from build123d import *

# Parameters (mm, degrees)
F0_R      = 16.5
F1_DEPTH  = 9.4
F2_R      = 14
F3_DEPTH  = 7.62
F4_R      = 2
F6_DEPTH  = 7
F8_DEPTH  = 5.5
F9_R      = 1
F10_R     = 10
F11_DEPTH = 3


with BuildPart() as f1:
    # F0 (on Top) → F1 (new body)
    with BuildSketch(Plane.XY):
        Circle(F0_R)
    extrude(amount=F1_DEPTH)

    # F2 (on face) → F3 (cut)
    with BuildSketch(Plane.XY.offset(9.4)):
        Circle(F2_R)
    extrude(amount=-F3_DEPTH, mode=Mode.SUBTRACT)

    # F4
    f4_edges = [f1.edges().sort_by_distance(p)[0] for p in [
        (-16.5, 0, 9.4),
    ]]
    fillet(f4_edges, radius=F4_R)

    # F5 (on face) → F6 (cut)
    with BuildSketch(Plane.XY.offset(9.4)):
        with BuildLine():
            ThreePointArc((-13.774977314, -2.5), (-14, 0), (-13.774977314, 2.5))
            Line((-13.774977314, 2.5), (-16.3095064303, 2.5))
            ThreePointArc((-16.3095064303, 2.5), (-16.5, 0), (-16.3095064303, -2.5))
            Line((-16.3095064303, -2.5), (-13.774977314, -2.5))
        make_face()
    extrude(amount=-F6_DEPTH, mode=Mode.SUBTRACT)

    # F7 (on face) → F8 (cut)
    with BuildSketch(Plane.XY.offset(9.4)):
        with BuildLine():
            ThreePointArc((-13.913931867, -1.55), (-14, 0), (-13.913931867, 1.55))
            Line((-13.913931867, 1.55), (-16.4270356425, 1.55))
            ThreePointArc((-16.4270356425, 1.55), (-16.5, 0), (-16.4270356425, -1.55))
            Line((-16.4270356425, -1.55), (-13.913931867, -1.55))
        make_face()
    extrude(amount=-F8_DEPTH, mode=Mode.SUBTRACT)

    # F9
    f9_edges = [f1.edges().sort_by_distance(p)[0] for p in [
        (-16.5, 0, 0),
    ]]
    fillet(f9_edges, radius=F9_R)

    # F10 (on face) → F11 (cut)
    with BuildSketch(Plane.XY.offset(1.78)):
        Circle(F10_R)
    extrude(amount=-F11_DEPTH, mode=Mode.SUBTRACT)


solid = f1.part
Input: part model. Units: mm. Frame: model coordinates. A direction names the side the tool comes from. Give positions to 0.01 mm unless a question says otherwise; leave off trailing zeros. Write each loop counter-clockwise with the first axis right and the second up, starting at its lowest first coordinate (ties: lowest second). Pieces come first, ordered by that corner, then holes. Notation, with made-up numbers: (9, 8.5) -> (42, 8.5) arc R13 ccw to (42, 26.5) -> close; hole circle Ø10 at (1.25, 79). An arc over 180 degrees is marked (long way). Use one line per item in the form item = value. Start each with the question number.
1) Section query A-A on y = 0. Return the cut outline in (x, z).
2) Section query C-C on z = 7. Return the cut outline in (x, y), then the cut area to 3 significant figures.
3) Draft query along Y for faces 4 (the cylindrical face through (15.738, 4.956, 4.155)), 5 (the flat face through (-2.1, 14, 9.4)), 6 (the flat face through (-15, -2.5, 6)). Return one class per face: pulls with the +Y half, pulls with the -Y half, needs draft (parallel to the pull), parting line crosses it, or undercut.
4) Pin query (flat end, axial travel): pin 1 (12 mm diameter, centred on x = -11.5, y = -11, fed in from -Z); pin 2 (1.4 mm diameter, centred on x = -14.5, y = 0.5, fed in from +Z); pin 3 (1 mm diameter, centred on y = 1.5, z = 4, fed in from -X); pin 4 (4 mm diameter, centred on y = -12.5, z = 3.5, fed in from -X). Return the tip coordinate at first contact, or that it passes through.
5) Ray query, probe 1 along Y at (x, z) = (0, 1.3); probe 2 along Z at (x, y) = (-8, 9); probe 3 along Y at (x, z) = (11.5, 2.5). Return the intervals inside material, ascending. Write a range as from..to.
6) Section query B-B on x = 0. Return the cut outline in (y, z), then the cut area to 3 significant figures.
7) Set-up query: faces 1 (the flat face through (3, -10, 0)), 2 (the flat face through (-3, 10, 1.78)), 3 (the flat face through (-15, 0, 2.4)). Return all of +Z, -Z, +X, -X, +Y, -Y with unobstructed straight access to the full face (end or side cutting, diameter ignored); none if empty.
Outcome:
q1.outline = (-16.5, 1) arc R1 ccw to (-15.5, 0) -> (-10, 0) -> (-10, 1.78) -> (-14, 1.78) -> (-14, 2.4) -> (-16.5, 2.4) -> close; (10, 0) -> (15.5, 0) arc R1 ccw to (16.5, 1) -> (16.5, 7.4) arc R2 ccw to (14.5, 9.4) -> (14, 9.4) -> (14, 1.78) -> (10, 1.78) -> close
q2.outline = (-16.31, -2.5) arc R16.5 ccw (long way) to (-16.31, 2.5) -> (-13.77, 2.5) arc R14 cw (long way) to (-13.77, -2.5) -> close
q2.area = 227 mm^2
q3.face_4 = parting line crosses it
q3.face_5 = needs draft
q3.face_6 = undercut
q4.pin_1 = 0
q4.pin_2 = 2.4
q4.pin_3 = 13.86
q4.pin_4 = -12.73
q5.probe_1 = -16.5..-10, 10..16.5
q5.probe_2 = 0..1.78
q5.probe_3 = -11.83..-7.98, 7.98..11.83
q6.outline = (-16.5, 1) arc R1 ccw to (-15.5, 0) -> (-10, 0) -> (-10, 1.78) -> (-14, 1.78) -> (-14, 9.4) -> (-14.5, 9.4) arc R2 ccw to (-16.5, 7.4) -> close; (10, 0) -> (15.5, 0) arc R1 ccw to (16.5, 1) -> (16.5, 7.4) arc R2 ccw to (14.5, 9.4) -> (14, 9.4) -> (14, 1.78) -> (10, 1.78) -> close
q6.area = 59.1 mm^2
q7.face_1 = -Z, +X, -X, +Y, -Y
q7.face_2 = +Z
q7.face_3 = +Z, -X
